Geometry check sheet. Reference: the model listing, model coordinates, mm. Round coordinates to 2 decimals unless told otherwise and drop trailing zeros. Write each loop counter-clockwise with the first axis right and the second up, starting at its lowest first coordinate (ties: lowest second). Pieces come first, ordered by that corner, then holes. Notation, with made-up numbers: (20.5, 51.25) -> (56.5, 51.25) arc R19 cw to (56.5, 67.25) -> close; hole circle Ø7 at (-37.75, -40). An arc over 180 degrees is marked (long way). Put each result on its own line as item: value. Start each with the question number.
from build123d import *

# Parameters (mm, degrees)
CYLINDER_R     = 2
CYLINDER_DEPTH = 5
BOX_W          = 10
BOX_H          = 5
BOX_DEPTH      = 5


with BuildPart() as cylinder:
    # Cylinder → Cylinder (new body)
    with BuildSketch(Plane(origin=(10, 5, 0), x_dir=(1, 0, 0), z_dir=(0, 0, 1))):
        Circle(CYLINDER_R)
    extrude(amount=CYLINDER_DEPTH)


with BuildPart() as cut:
    # Box → Box (new body)
    with BuildSketch(Plane.XY):
        with Locations((5, 2.5)):
            Rectangle(BOX_W, BOX_H)
    extrude(amount=BOX_DEPTH)

    # Cut: cut Cylinder
    add(cylinder.part, mode=Mode.SUBTRACT)


solid = cut.part
(1) Material ranges on L1, parallel to X at y = 4.55, z = 4.05; L2, parallel to Y at x = 8.5, z = 1.9; L3, parallel to X at y = 4.2, z = 3.95, recorded low to high. Write a range as from..to.
(2) Sectioned sample at B-B (y = 3.25). Record the cut outline in (x, z).
(3) Sectioned sample at C-C (x = 9.5). Record the cut outline in (y, z), and give its area (3 significant figures).
(4) Sectioned sample at A-A (z = 0.4). Record the cut outline in (x, y), and give its area (3 significant figures).
Found:
1. L1: 0..8.05
1. L2: 0..3.68
1. L3: 0..8.17
2. outline: (0, 0) -> (9.03, 0) -> (9.03, 5) -> (0, 5) -> close
3. outline: (0, 0) -> (3.06, 0) -> (3.06, 5) -> (0, 5) -> close
3. area: 15.3 mm2
4. outline: (0, 0) -> (10, 0) -> (10, 3) arc R2 cw to (8, 5) -> (0, 5) -> close
4. area: 46.9 mm2
